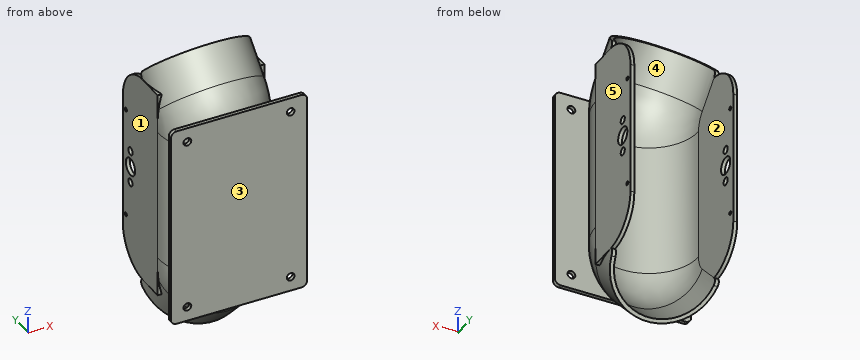
```python
from build123d import *

# Parameters (mm, degrees)
SKETCH6_W           = 70
SKETCH6_H           = 105
BOSS_EXTRUDE1_DEPTH = 2
CUT_EXTRUDE1_START  = -25.4
SKETCH4_R           = 2
CUT_EXTRUDE1_DEPTH  = 5
FILLET1_R           = 3
FILLET2_R           = 3
BOSS_EXTRUDE2_REACH = 105.819
SKETCH9_W           = 2
SKETCH9_H           = 109.10689276
SKETCH10_R          = 2
SKETCH10_R_2        = 4.5
CUT_EXTRUDE2_DEPTH  = 105.083069428
SKETCH11_R          = 1
CUT_EXTRUDE4_DEPTH  = 105.083069428
FILLET4_R           = 20


with BuildPart() as part:
    # Sweep2: sweep along a path in Sketch3
    with BuildLine(Plane(origin=(0, 0, 0), x_dir=(0, 0, -1), z_dir=(1, 0, 0))) as sweep2_path:
        Line((76.2, -2.212849708), (62.515728753, -15.897120955))
        ThreePointArc((62.515728753, -15.897120955), (49.5387948, -24.568031008), (34.231457505, -27.612849708))
        Line((34.231457505, -27.612849708), (-34.231457505, -27.612849708))
        ThreePointArc((-34.231457505, -27.612849708), (-49.5387948, -24.568031008), (-62.515728753, -15.897120955))
        Line((-62.515728753, -15.897120955), (-76.2, -2.212849708))
    # Sketch1 → Sweep2 (sweep)
    with BuildSketch(Plane.XY):
        with BuildLine():
            Line((-25.4, 0), (-27.4, 0))
            ThreePointArc((-27.4, 0), (0, -27.4), (27.4, 0))
            Line((27.4, 0), (25.4, 0))
            ThreePointArc((25.4, 0), (0, -25.4), (-25.4, 0))
        make_face()
    sweep(path=sweep2_path.line)

    # Sketch6 → Boss-Extrude1 (add)
    with BuildSketch(Plane(origin=(0, -27.4, 0), x_dir=(-1, 0, 0), z_dir=(0, -1, 0))):
        Rectangle(SKETCH6_W, SKETCH6_H)
    extrude(amount=-BOSS_EXTRUDE1_DEPTH)

    # Sketch4 → Cut-Extrude1 (cut)
    with BuildSketch(Plane(origin=(0, 0, 0), x_dir=(1, 0, 0), z_dir=(0, 1, 0)).offset(CUT_EXTRUDE1_START)):
        with Locations(Location((-26.5, 45, 0), (0, 0, 90))):
            Circle(SKETCH4_R)
        with Locations(Location((26.5, 45, 0), (0, 0, 90))):
            Circle(SKETCH4_R)
        with Locations(Location((-26.5, -45, 0), (0, 0, 90))):
            Circle(SKETCH4_R)
        with Locations(Location((26.5, -45, 0), (0, 0, 90))):
            Circle(SKETCH4_R)
    extrude(amount=-CUT_EXTRUDE1_DEPTH, mode=Mode.SUBTRACT)

    # Fillet1
    fillet1_edges = [part.edges().sort_by_distance(p)[0] for p in [
        (26.4, 17.312383569, 56.674766724),
        (26.4, 17.312383569, -56.674766724),
        (-26.4, 17.312383569, -56.674766724),
        (-26.4, 17.312383569, 56.674766724),
    ]]
    fillet(fillet1_edges, radius=FILLET1_R)

    # Fillet2
    fillet2_edges = [part.edges().sort_by_distance(p)[0] for p in [
        (35, -26.4, 52.5),
        (35, -26.4, -52.5),
        (-35, -26.4, -52.5),
        (-35, -26.4, 52.5),
    ]]
    fillet(fillet2_edges, radius=FILLET2_R)

    # Boss-Extrude2: up to this face of the body (flat: up to its plane)
    boss_extrude2_end = Plane(part.part.faces().sort_by_distance((-26.4, 0, 0))[0])
    # Sketch9 → Boss-Extrude2 (add, up to the picked face)
    with BuildSketch(Plane(origin=(0, 34, 0), x_dir=(1, 0, 0), z_dir=(0, 1, 0)), mode=Mode.PRIVATE) as boss_extrude2_sk1:
        with Locations((-26.4, 0)):
            Rectangle(SKETCH9_W, SKETCH9_H)
    boss_extrude2_tool1 = split(extrude(boss_extrude2_sk1.sketch, amount=-BOSS_EXTRUDE2_REACH, mode=Mode.PRIVATE), bisect_by=boss_extrude2_end, keep=Keep.BOTH, mode=Mode.PRIVATE)
    # Sketch9 → Boss-Extrude2 (add, up to the picked face)
    with BuildSketch(Plane(origin=(0, 34, 0), x_dir=(1, 0, 0), z_dir=(0, 1, 0)), mode=Mode.PRIVATE) as boss_extrude2_sk2:
        with Locations((26.4, 0)):
            Rectangle(SKETCH9_W, SKETCH9_H)
    boss_extrude2_tool2 = split(extrude(boss_extrude2_sk2.sketch, amount=-BOSS_EXTRUDE2_REACH, mode=Mode.PRIVATE), bisect_by=boss_extrude2_end, keep=Keep.BOTH, mode=Mode.PRIVATE)
    add(boss_extrude2_tool1.solids().sort_by(Axis((-26.4, 34, 0), (0, -1, 0)))[0])
    add(boss_extrude2_tool2.solids().sort_by(Axis((26.4, 34, 0), (0, -1, 0)))[0])

    # Sketch10 → Cut-Extrude2 (cut, through all)
    with BuildSketch(Plane.ZY.offset(27.4)):
        with Locations((-8.55, 26.5)):
            Circle(SKETCH10_R)
        with Locations((8.55, 26.5)):
            Circle(SKETCH10_R)
        with Locations((0, 26.5)):
            Circle(SKETCH10_R_2)
    extrude(amount=-CUT_EXTRUDE2_DEPTH, mode=Mode.SUBTRACT)

    # Sketch11 → Cut-Extrude4 (cut, through all)
    with BuildSketch(Plane.ZY.offset(27.4)):
        with Locations((-28.55, 31)):
            Circle(SKETCH11_R)
        with Locations((28.55, 31)):
            Circle(SKETCH11_R)
    extrude(amount=-CUT_EXTRUDE4_DEPTH, mode=Mode.SUBTRACT)

    # Fillet4
    # the kernel refuses this fillet: 20 mm, written as the material it takes off along each edge
    with BuildSketch(Plane(origin=(77.311256771, 34, 54.55344638), x_dir=(0, 0, -1), z_dir=(-1, 0, 0)), Plane(origin=(24.511256771, 34, 54.55344638), x_dir=(0, 0, -1), z_dir=(-1, 0, 0)), Plane(origin=(-24.511256771, 34, -54.55344638), x_dir=(0, 0, 1), z_dir=(1, 0, 0)), Plane(origin=(-77.311256771, 34, -54.55344638), x_dir=(0, 0, 1), z_dir=(1, 0, 0))) as fillet4_piece_1:
        with BuildLine():
            CenterArc((19.964502708, 20), FILLET4_R, 183.414164929, 86.585835071)
            Line((0, 18.808936775), (0, 0))
            Line((0, 0), (19.964502708, 0))
        make_face()
    extrude(amount=101.822513542, mode=Mode.SUBTRACT)


solid = part.part
```
Model file for the job. Use its own axes, mm. Face numbers are marked on the shaded views. A direction names the side the tool comes from. Round coordinates to 2 decimals unless told otherwise and drop trailing zeros. Write each loop counter-clockwise with the first axis right and the second up, starting at its lowest first coordinate (ties: lowest second). Pieces come first, ordered by that corner, then holes. Notation, with made-up numbers: (41.5, 85) - (46.5, 85) arc R18 ccw to (46.5, 115) - close; hole circle Ø4 at (-39, -17). An arc over 180 degrees is marked (long way). Use CSV: the item, a comma, the result in double quotes. Start each with the question number.
Item 1: Pin check, flat tips, straight feed: P1, Ø2, axis at y = -1, z = 35, coming from the -X side; P2, Ø6.5, axis at x = 26.5, z = 45, coming from the -Y side; P3, Ø0.6, axis at x = 14, y = -26.5, coming from the +Z side; P4, Ø3, axis at x = -6.5, z = -39, coming from the +Y side. Stop position of each tip, or through.
Item 2: Band-saw the part on C-C (x = -30). Write the cut outline in (y, z).
Item 3: Two-plate mould, pull along Z, no slides. Class the marked faces 4 and 5: released by +Z, released by -Z, zero draft, split by the parting line, or undercut.
Item 4: Band-saw the part on A-A (z = -8.55). Write the cut outline in (x, y).
Item 5: Drill centre lines: L1, parallel to Z at x = -26.5, y = -26.9; L2, parallel to X at y = 10, z = 3.5; L3, parallel to Z at x = -9.5, y = -21. Where is each one in solid material? Low to high. Write a range as [from, to].
Item 6: Band-saw the part on B-B (y = 26.5). State how many separate pieces and enclosed holes the cut face has, and give its area (3 significant figures).
Item 7: Tool access for the marked faces 1, 2 and 3: list every direction of +Z, -Z, +X, -X, +Y, -Y with a clear straight run to the whole face (end or side of a thin tool).
Checked values:
1,P1,"stops at x = -27.4"
1,P2,"stops at y = -27.4"
1,P3,"stops at z = 52.5"
1,P4,"stops at y = -23.75"
2,outline,"(-27.4, -52.5) - (-25.4, -52.5) - (-25.4, 52.5) - (-27.4, 52.5) - close"
3,face 4,"undercut"
3,face 5,"zero draft"
4,outline,"(-35, -27.4) - (35, -27.4) - (35, -25.4) - (10.28, -25.4) arc R27.4 ccw to (27.4, 0) - (27.4, 24.5) - (25.4, 24.5) - (25.4, 0) arc R25.4 cw to (-25.4, 0) - (-25.4, 24.5) - (-27.4, 24.5) - (-27.4, 0) arc R27.4 ccw to (-10.28, -25.4) - (-35, -25.4) - close; (-27.4, 28.5) - (-25.4, 28.5) - (-25.4, 34) - (-27.4, 34) - close; (25.4, 28.5) - (27.4, 28.5) - (27.4, 34) - (25.4, 34) - close"
5,L1,"z = [-52.5, -47], [-43, 43], [47, 52.5]"
5,L2,"x = [-27.4, -25.4], [25.4, 27.4]"
5,L3,"z = [-52.56, -47.54], [47.54, 52.56]"
6,separate pieces,"8"
6,enclosed holes,"0"
6,area,"334 mm²"
7,face 1,"+Z, -Z, -X, +Y"
7,face 2,"+Y"
7,face 3,"+Z, -Z, +X, -X, -Y"
